Can you work these out from the model? Positions are in its coordinate system, mm. Give positions to 0.01 mm unless a question says otherwise; leave off trailing zeros. Loops run counter-clockwise (first coordinate to the right, second up) from the corner with the lowest first, then second, coordinate; pieces in that order, holes last. Notation, with made-up numbers: (11, 85) -> (29, 85) arc R17 ccw to (29, 98) -> close; hole circle Ø6 at (77.5, 20). An arc over 180 degrees is marked (long way). Use CSV: the item, a comma, the result in double quotes.
from build123d import *

# Parameters (mm, degrees)
F0_R     = 4.191
F1_DEPTH = 1.905


with BuildPart() as f1:
    # F0 (on Right) → F1 (new body)
    with BuildSketch(Plane.YZ):
        with BuildLine():
            Line((9.525, 0), (7.910989, 19.698203))
            ThreePointArc((7.910989, 19.698203), (0, 26.9875), (-7.910989, 19.698203))
            Line((-7.910989, 19.698203), (-9.525, 0))
            Line((-9.525, 0), (9.525, 0))
        make_face()
        with Locations((0, 19.05)):
            Circle(F0_R, mode=Mode.SUBTRACT)
    extrude(amount=F1_DEPTH)


solid = f1.part
(1) If we section it at C-C, the plane z = 19.05: Write out the boundary of the cut face in (x, y) (3 decimals), then the cut area to 3 significant figures.
Answer sheet:
outline,"(0, -7.964) -> (1.905, -7.964) -> (1.905, -4.191) -> (0, -4.191) -> close; (0, 4.191) -> (1.905, 4.191) -> (1.905, 7.964) -> (0, 7.964) -> close"
area,"14.4 mm2"
(2) If I drill on L1, parallel to Y at x = 0.95, z = 22; L2, parallel to Y at x = 0.2, z = 2; L3, parallel to Z at x = 0.3, y = 6.25, over which ranges is the centre line in solid material (lowest first)? Write a range as from..to.
Answer sheet:
L1,"y = -7.37..-2.98, 2.98..7.37"
L2,"y = -9.36..9.36"
L3,"z = 0..23.94"
(3) If we section it at A-A, the plane y = 0: Write out the boundary of the cut face in (x, z) (1 decimal).
Answer sheet:
outline,"(0, 0) -> (1.9, 0) -> (1.9, 14.9) -> (0, 14.9) -> close; (0, 23.2) -> (1.9, 23.2) -> (1.9, 27) -> (0, 27) -> close"
(4) If we section it at D-D, the plane y = 5.25: Write out the boundary of the cut face in (x, z) (3 decimals).
Answer sheet:
outline,"(0, 0) -> (1.905, 0) -> (1.905, 25.003) -> (0, 25.003) -> close"
(5) Will this pin go through, and if not, where does the flat tip stop? pin 1 Ø7.5 at (y, z) = (0, 19.05) entering from -X.
Answer sheet:
pin 1,"passes through"
(6) We'd pull the mould along Z, two halves only. Please class faces 1 (the face through (1.905, 0, 11)), 2 (the face through (0.94, -0.91, 14.96)), 3 (the face through (0.94, 8.73, 9.71)), 4 (the face through (1, 0, 0)): released by +Z, released by -Z, zero draft, split by the parting line, or undercut.
Answer sheet:
face 1,"zero draft"
face 2,"undercut"
face 3,"released by +Z"
face 4,"released by -Z"
